```python
from build123d import *

# Parameters (mm, degrees)
BOSS_EXTRUDE1_DEPTH  = 20
SKETCH3_OUTSIDE_W    = 88.614
SKETCH3_OUTSIDE_H    = 38.614
CUT_EXTRUDE2_DEPTH   = 57.789083458
BOSS_EXTRUDE3_START  = 20
SKETCH4_R            = 10
BOSS_EXTRUDE3_DEPTH  = 225
BOSS_EXTRUDE22_DEPTH = 6
SKETCH47_R           = 12.424441969
CUT_EXTRUDE8_DEPTH   = 212.778185845


with BuildPart() as part:
    # Sketch2 → Boss-Extrude1 (new body)
    with BuildSketch(Plane(origin=(0, 0, 0), x_dir=(1, 0, 0), z_dir=(0, 1, 0))):
        with BuildLine():
            Line((-35, -14), (-35, 14))
            ThreePointArc((-35, 14), (-33.242640687, 18.242640687), (-29, 20))
            Line((-29, 20), (8.717414306, 20))
            ThreePointArc((8.717414306, 20), (9.971663529, 19.867440574), (11.1704919, 19.475619629))
            Line((11.1704919, 19.475619629), (30.270770125, 10.918694984))
            ThreePointArc((30.270770125, 10.918694984), (33.714393532, 7.967227328), (35, 3.617868812))
            Line((35, 3.617868812), (35, -3.617868812))
            ThreePointArc((35, -3.617868812), (33.714393532, -7.967227328), (30.270770125, -10.918694984))
            Line((30.270770125, -10.918694984), (11.1704919, -19.475619629))
            ThreePointArc((11.1704919, -19.475619629), (9.971663529, -19.867440574), (8.717414306, -20))
            Line((8.717414306, -20), (-29, -20))
            ThreePointArc((-29, -20), (-33.242640687, -18.242640687), (-35, -14))
        make_face()
    extrude(amount=BOSS_EXTRUDE1_DEPTH)

    # Sketch3 outside → Cut-Extrude2 (cut, through all)
    with BuildSketch(Plane.XY.offset(20)):
        with Locations((0, 10)):
            Rectangle(SKETCH3_OUTSIDE_W, SKETCH3_OUTSIDE_H)
        with BuildLine():
            Line((-35, 20), (-23.9, 20))
            ThreePointArc((-23.9, 20), (-12.33766892, 12.25), (-0.77533784, 20))
            Line((-0.77533784, 20), (35, 20))
            Line((35, 20), (35, 16))
            Line((35, 16), (1.651165913, 16))
            ThreePointArc((1.651165913, 16), (-12.33766892, 8.25), (-26.326503754, 16))
            Line((-26.326503754, 16), (-35, 16))
            Line((-35, 16), (-35, 20))
        make_face(mode=Mode.SUBTRACT)
    extrude(amount=-CUT_EXTRUDE2_DEPTH, mode=Mode.SUBTRACT)



with BuildPart() as body_2:
    # Sketch4 → Boss-Extrude3 (new body)
    with BuildSketch(Plane(origin=(0, 0, 0), x_dir=(1, 0, 0), z_dir=(0, 1, 0)).offset(BOSS_EXTRUDE3_START)):
        with Locations(Location((19.22466216, 0, 0), (0, 0, 90))):
            Circle(SKETCH4_R)
    extrude(amount=-BOSS_EXTRUDE3_DEPTH)


with BuildPart() as part_1:
    add(part.part)

    add(body_2.part)  # Boss-Extrude22 merges body 2
    # Sketch46 → Boss-Extrude22 (add)
    with BuildSketch(Plane(origin=(0, 20, 0), x_dir=(1, 0, 0), z_dir=(0, 1, 0))):
        with BuildLine():
            Line((8.717414306, 20), (-29, 20))
            ThreePointArc((-29, 20), (-33.242640687, 18.242640687), (-35, 14))
            Line((-35, 14), (-35, -14))
            ThreePointArc((-35, -14), (-33.242640687, -18.242640687), (-29, -20))
            Line((-29, -20), (8.717414306, -20))
            ThreePointArc((8.717414306, -20), (9.971663529, -19.867440574), (11.1704919, -19.475619629))
            Line((11.1704919, -19.475619629), (30.270770125, -10.918694984))
            ThreePointArc((30.270770125, -10.918694984), (33.714393532, -7.967227328), (35, -3.617868812))
            Line((35, -3.617868812), (35, 3.617868812))
            ThreePointArc((35, 3.617868812), (33.714393532, 7.967227328), (30.270770125, 10.918694984))
            Line((30.270770125, 10.918694984), (11.1704919, 19.475619629))
            ThreePointArc((11.1704919, 19.475619629), (9.971663529, 19.867440574), (8.717414306, 20))
        make_face()
    extrude(amount=BOSS_EXTRUDE22_DEPTH)

    # Sketch47 → Cut-Extrude8 (cut, through all)
    with BuildSketch(Plane.XY.offset(20)):
        with Locations((-12.32630139, 24.675301972)):
            Circle(SKETCH47_R)
    extrude(amount=-CUT_EXTRUDE8_DEPTH, mode=Mode.SUBTRACT)


solid = part_1.part
```
Input: part model. Units: mm. Frame: model coordinates. A direction names the side the tool comes from. Round coordinates to 2 decimals unless told otherwise and drop trailing zeros. Loops run counter-clockwise (first coordinate to the right, second up) from the corner with the lowest first, then second, coordinate; pieces in that order, holes last. Notation, with made-up numbers: M -12.75,14 L -4.75,14 A32 cw -4.75,48 Z; hole C 55,36.5 d2. An arc over 180 degrees is marked long. Answer in a Markdown table with one row per item. Add a question column.
1. Section D-D (x = -21.5). Output: boundary loops of the cut face in (y, z).
2. Set-up query: faces 1 (the face through (-31, 16, 0)), 2 (the face through (-0.029, 22.905, 0.28)), 3 (the face through (9.31, -92.95, 1.3)), 4 (the face through (19, -205, 0)). Return all of +Z, -Z, +X, -X, +Y, -Y with unobstructed straight access to the full face (end or side cutting, diameter ignored); none if empty.
3. Mould query, pull axis X, two halves, no side actions, for faces 5 (the face through (7, 16, 0)), 6 (the face through (-6, 13, 20)), 7 (the face through (-12.54, 12.25, 0.28)), 8 (the face through (-33.196, 20.93, -18.289)). Classes: released by +X, released by -X, zero draft, split by the parting line, or undercut.
4. Contact query for flat-ended pins moving along their axis: pin 1 (4.5 mm diameter, centred on x = -31, z = -8, fed in from -Y); pin 2 (10 mm diameter, centred on x = 6, y = -146, fed in from -Z); pin 3 (6 mm diameter, centred on x = -11.5, z = -14.5, fed in from +Y). Output: stop coordinate, or through.
5. Section C-C (y = -171.5). Output: boundary loops of the cut face in (x, z).
6. Ray query, probe 1 along Y at (x, z) = (6, -17); probe 2 along X at (y, z) = (-100, 0.5); probe 3 along Y at (x, z) = (-5.5, 11). Return the intervals inside material, ascending.
7. Section B-B (x = 4). Output: boundary loops of the cut face in (y, z), and give its area (3 significant figures).
Values follow:
| question | item | result |
|---|---|---|
| 1 | outline | M 11.03,-20 L 16.25,-20 L 16.25,20 L 11.03,20 Z |
| 2 | face 1 | +Z, -Z, -X, -Y |
| 2 | face 2 | +Z, -Z |
| 2 | face 3 | -Y |
| 2 | face 4 | +Z, -Z, +X, -X, -Y |
| 3 | face 5 | undercut |
| 3 | face 6 | zero draft |
| 3 | face 7 | undercut |
| 3 | face 8 | released by -X |
| 4 | pin 1 | y = 16 |
| 4 | pin 2 | z = -5.69 |
| 4 | pin 3 | y = 12.85 |
| 5 | outline | C 19.22,0 d20 |
| 6 | probe 1 | 16 to 26 |
| 6 | probe 2 | 9.24 to 29.21 |
| 6 | probe 3 | 9.73 to 14.29 |
| 7 | outline | M 16,-20 L 26,-20 L 26,20 L 16,20 Z |
| 7 | area | 400 mm^2 |
